Read the model definition and answer for the solid it produces. Units are mm, in the model's axes. Face numbers are marked on the shaded views. Coordinates: 2 decimals unless noted, no trailing zeros. Write each loop counter-clockwise with the first axis right and the second up, starting at its lowest first coordinate (ties: lowest second). Pieces come first, ordered by that corner, then holes.
1) Find the intervals of material crossed by line 1 (Y direction, x = -23.25, z = 10.5); line 2 (X direction, y = 33.5, z = 0); line 3 (Z direction, x = -7.5, y = 38.5), in increasing order.
2) The part is cut by section D-D (x = 0). Determine the outline of the cut face in (y, z).
3) Determine the mould class of the marked faces 1, 2, 3 and 4 for opening direction X: +X half, -X half, draft (parallel to the pull), parting line (faces both ways), or undercut.
4) Each of these flat-tipped pins is pushed along its axis until it touches: pin 1 Ø3.5 at (y, z) = (6.5, 10.5) entering from -X; pin 2 Ø4.5 at (x, y) = (-0.04, 34.93) entering from +Z. Where does it stop, or does it pass through?
5) The part is cut by section A-A (z = 10.5). Determine the outline of the cut face in (x, y).
6) The part is cut by section C-C (y = 24). Determine the outline of the cut face in (x, z), then the cut area to 3 significant figures.
7) The part is cut by section B-B (z = -5). Determine the outline of the cut face in (x, y).
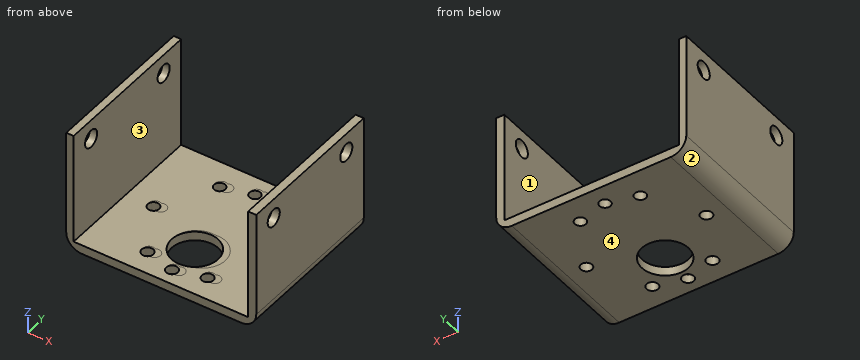
from build123d import *

# Parameters (mm, degrees)
BOSS_EXTRUDE1_DEPTH = 40
FILLET1_R           = 4
SKETCH2_R           = 1.5
SKETCH2_R_2         = 6
CUT_EXTRUDE1_DEPTH  = 40
SKETCH3_R           = 2.25
CUT_EXTRUDE2_DEPTH  = 76
SKETCH4_R           = 1.5
SKETCH4_R_2         = 6
BOSS_EXTRUDE2_DEPTH = 2.346753
SKETCH5_R           = 1.5
SKETCH5_R_2         = 6
CUT_EXTRUDE3_DEPTH  = 10
SKETCH7_W           = 0.19
SKETCH7_H           = 28.653247295
CUT_EXTRUDE4_DEPTH  = 463
SKETCH11_R          = 6
BOSS_EXTRUDE3_DEPTH = 2.346753
SKETCH12_R          = 6
CUT_EXTRUDE7_DEPTH  = 10
SKETCH13_R          = 1.5
BOSS_EXTRUDE4_DEPTH = 2.346753
SKETCH14_R          = 1.475604419
SKETCH14_R_2        = 1.463203764
SKETCH14_R_3        = 1.5
SKETCH14_R_4        = 1.434937512
SKETCH14_R_5        = 1.505191791
SKETCH14_R_6        = 1.44518411
CUT_EXTRUDE8_DEPTH  = 10


with BuildPart() as part:
    # Sketch1 → Boss-Extrude1 (new body)
    with BuildSketch(Plane(origin=(0, 0, 0), x_dir=(1, 0, 0), z_dir=(0, 1, 0))):
        Polygon((-22.403304398, -15.5), (-22.403304398, 13.153247295), (22.214170378, 13.153247295), (22.214170378, -15.5), (24.5, -15.5), (24.5, 15.5), (-24.5, 15.5), (-24.5, -15.5), align=None)
    extrude(amount=BOSS_EXTRUDE1_DEPTH)

    # Fillet1
    fillet1_edges = [part.edges().sort_by_distance(p)[0] for p in [
        (-24.5, 20, -15.5),
        (24.5, 20, -15.5),
    ]]
    fillet(fillet1_edges, radius=FILLET1_R)

    # Sketch2 → Cut-Extrude1 (cut)
    with BuildSketch(Plane(origin=(0, 0, -15.5), x_dir=(-1, 0, 0), z_dir=(0, 0, -1))):
        with Locations((14, 20)):
            Circle(SKETCH2_R)
        with Locations((-17, 20)):
            Circle(SKETCH2_R)
        with Locations((-1.5, 4.5)):
            Circle(SKETCH2_R)
        with Locations((-1.5, 35.5)):
            Circle(SKETCH2_R)
        with Locations((-9.25, 6.576606241)):
            Circle(SKETCH2_R)
        with Locations((-9.25, 33.423393759)):
            Circle(SKETCH2_R)
        with Locations((6.25, 33.423393759)):
            Circle(SKETCH2_R)
        with Locations((6.25, 6.576606241)):
            Circle(SKETCH2_R)
        with Locations((-1.5, 13)):
            Circle(SKETCH2_R_2)
    extrude(amount=-CUT_EXTRUDE1_DEPTH, mode=Mode.SUBTRACT)

    # Sketch3 → Cut-Extrude2 (cut)
    with BuildSketch(Plane.ZY.offset(24.5)):
        with Locations((10.5, 6.5)):
            Circle(SKETCH3_R)
        with Locations((10.5, 33.5)):
            Circle(SKETCH3_R)
    extrude(amount=-CUT_EXTRUDE2_DEPTH, mode=Mode.SUBTRACT)

    # Sketch4 → Boss-Extrude2 (add)
    with BuildSketch(Plane(origin=(0, 0, -15.5), x_dir=(-1, 0, 0), z_dir=(0, 0, -1))):
        with Locations((6.25, 33.423393759)):
            Circle(SKETCH4_R)
        with Locations((14, 20)):
            Circle(SKETCH4_R)
        with Locations((6.25, 6.576606241)):
            Circle(SKETCH4_R)
        with Locations((-1.5, 4.5)):
            Circle(SKETCH4_R)
        with Locations((-9.25, 6.576606241)):
            Circle(SKETCH4_R)
        with Locations((-17, 20)):
            Circle(SKETCH4_R)
        with Locations((-1.5, 35.5)):
            Circle(SKETCH4_R)
        with Locations((-9.25, 33.423393759)):
            Circle(SKETCH4_R)
        with Locations((-1.5, 13)):
            Circle(SKETCH4_R_2)
    extrude(amount=-BOSS_EXTRUDE2_DEPTH)

    # Sketch5 → Cut-Extrude3 (cut)
    with BuildSketch(Plane(origin=(0, 0, -15.5), x_dir=(-1, 0, 0), z_dir=(0, 0, -1))):
        with Locations((15.5, 20)):
            Circle(SKETCH5_R)
        with Locations((0, 4.5)):
            Circle(SKETCH5_R)
        with Locations((-15.5, 20)):
            Circle(SKETCH5_R)
        with Locations((0, 35.5)):
            Circle(SKETCH5_R)
        with Locations((7.75, 33.423393759)):
            Circle(SKETCH5_R)
        with Locations((-7.75, 33.423393759)):
            Circle(SKETCH5_R)
        with Locations((-7.75, 6.576606241)):
            Circle(SKETCH5_R)
        with Locations((7.75, 6.576606241)):
            Circle(SKETCH5_R)
        with Locations((0, 13)):
            Circle(SKETCH5_R_2)
    extrude(amount=-CUT_EXTRUDE3_DEPTH, mode=Mode.SUBTRACT)

    # Sketch7 → Cut-Extrude4 (cut)
    with BuildSketch(Plane.XZ):
        with Locations((-22.498304398, 1.173376353)):
            Rectangle(SKETCH7_W, SKETCH7_H)
        with Locations((22.309170378, 1.173376353)):
            Rectangle(SKETCH7_W, SKETCH7_H)
    extrude(amount=-CUT_EXTRUDE4_DEPTH, mode=Mode.SUBTRACT)

    # Sketch11 → Boss-Extrude3 (add)
    with BuildSketch(Plane(origin=(0, 0, -15.5), x_dir=(-1, 0, 0), z_dir=(0, 0, -1))):
        with Locations((0, 13)):
            Circle(SKETCH11_R)
    extrude(amount=-BOSS_EXTRUDE3_DEPTH)

    # Sketch12 → Cut-Extrude7 (cut)
    with BuildSketch(Plane(origin=(0, 0, -15.5), x_dir=(-1, 0, 0), z_dir=(0, 0, -1))):
        with Locations((0, 12.5)):
            Circle(SKETCH12_R)
    extrude(amount=-CUT_EXTRUDE7_DEPTH, mode=Mode.SUBTRACT)

    # Sketch13 → Boss-Extrude4 (add)
    with BuildSketch(Plane(origin=(0, 0, -15.5), x_dir=(-1, 0, 0), z_dir=(0, 0, -1))):
        with Locations((7.75, 6.576606241)):
            Circle(SKETCH13_R)
        with Locations((0, 4.5)):
            Circle(SKETCH13_R)
        with Locations((-7.75, 6.576606241)):
            Circle(SKETCH13_R)
        with Locations((-15.5, 20)):
            Circle(SKETCH13_R)
        with Locations((-7.75, 33.423393759)):
            Circle(SKETCH13_R)
        with Locations((0, 35.5)):
            Circle(SKETCH13_R)
        with Locations((7.75, 33.423393759)):
            Circle(SKETCH13_R)
        with Locations((15.5, 20)):
            Circle(SKETCH13_R)
    extrude(amount=-BOSS_EXTRUDE4_DEPTH)

    # Sketch14 → Cut-Extrude8 (cut)
    with BuildSketch(Plane(origin=(0, 0, -15.5), x_dir=(-1, 0, 0), z_dir=(0, 0, -1))):
        with Locations((15.475197646, 19.465354549)):
            Circle(SKETCH14_R)
        with Locations((-15.475197646, 19.465354549)):
            Circle(SKETCH14_R_2)
        with Locations((0, 3.990156903)):
            Circle(SKETCH14_R_3)
        with Locations((0.042141816, 34.934937512)):
            Circle(SKETCH14_R_4)
        with Locations((7.752595896, 6.072110018)):
            Circle(SKETCH14_R_5)
        with Locations((-7.752600927, 6.072112931)):
            Circle(SKETCH14_R_3)
        with Locations((-7.722592055, 32.875921806)):
            Circle(SKETCH14_R_6)
        with Locations((7.722592055, 32.875921806)):
            Circle(SKETCH14_R_6)
    extrude(amount=-CUT_EXTRUDE8_DEPTH, mode=Mode.SUBTRACT)


solid = part.part
Reported:
1. line 1: y = 0 to 4.25, 8.75 to 31.25, 35.75 to 40
1. line 2: x = -24.5 to -22.59, 22.4 to 24.5
1. line 3: z = -15.5 to -13.15
2. outline: (0, -15.5) - (2.49, -15.5) - (2.49, -13.15) - (0, -13.15) - close; (5.49, -15.5) - (6.5, -15.5) - (6.5, -13.15) - (5.49, -13.15) - close; (18.5, -15.5) - (33.5, -15.5) - (33.5, -13.15) - (18.5, -13.15) - close; (36.37, -15.5) - (40, -15.5) - (40, -13.15) - (36.37, -13.15) - close
3. face 1: undercut
3. face 2: -X half
3. face 3: undercut
3. face 4: draft
4. pin 1: passes through
4. pin 2: stops at z = -13.15
5. outline: (-24.5, 0) - (-22.59, 0) - (-22.59, 4.25) - (-24.5, 4.25) - close; (-24.5, 8.75) - (-22.59, 8.75) - (-22.59, 31.25) - (-24.5, 31.25) - close; (-24.5, 35.75) - (-22.59, 35.75) - (-22.59, 40) - (-24.5, 40) - close; (22.4, 0) - (24.5, 0) - (24.5, 4.25) - (22.4, 4.25) - close; (22.4, 8.75) - (24.5, 8.75) - (24.5, 31.25) - (22.4, 31.25) - close; (22.4, 35.75) - (24.5, 35.75) - (24.5, 40) - (22.4, 40) - close
6. outline: (-24.5, -11.5) arc R4 ccw to (-20.5, -15.5) - (20.5, -15.5) arc R4 ccw to (24.5, -11.5) - (24.5, 15.5) - (22.4, 15.5) - (22.4, -13.15) - (-22.59, -13.15) - (-22.59, 15.5) - (-24.5, 15.5) - close
6. area: 223 mm2
7. outline: (-24.5, 0) - (-22.59, 0) - (-22.59, 40) - (-24.5, 40) - close; (22.4, 0) - (24.5, 0) - (24.5, 40) - (22.4, 40) - close
